Build history of the part. All positions in model axes, mm. Face numbers are marked on the shaded views. A direction names the side the tool comes from. Give positions to 0.01 mm unless a question says otherwise; leave off trailing zeros. Loops run counter-clockwise (first coordinate to the right, second up) from the corner with the lowest first, then second, coordinate; pieces in that order, holes last. Notation, with made-up numbers: (58, 38.5) -> (88, 38.5) arc R12 cw to (88, 43.5) -> close; hole circle Ø6 at (50.5, 82.5). An arc over 180 degrees is marked (long way). One line per question, with ' | ' between items. Start each with the question number.
(1) Slice it at A-A, the plane y = 0. Write the cut outline in (x, z), then the cut area to 4 significant figures.
(2) Slice it at C-C, the plane y = -3.75. Write the cut outline in (x, z), then the cut area to 4 significant figures.
(3) Flat gauge pins, fed straight in: pin 1 Ø3 at (y, z) = (0.5, 6) entering from -X; pin 2 Ø5.5 at (x, y) = (0, 0) entering from +Z; pin 3 Ø5 at (x, z) = (3.5, 12) entering from +Y; pin 4 Ø4 at (x, y) = (-3, 2) entering from +Z. Where does each tip first touch, or does it go through?
(4) Slice it at D-D, the plane z = 12.75. Write the cut outline in (x, y).
(5) Drill centre lines: L1, parallel to Y at x = 0, z = 0.35; L2, parallel to X at y = -4, z = 10.5; L3, parallel to Z at x = 3.5, y = 4.25. Where is each one in solid material? Low to high. Write a range as from..to.
(6) Mould opens along Y. For the marked faces 3, 4 and 5 say: pulls with the +Y half, pulls with the -Y half, needs draft (parallel to the pull), parting line crosses it, or undercut.
(7) 3-axis set-ups, long thin cutter, end or side, ignore diameter. For the marked faces 1 and 2: which of +Z, -Z, +X, -X, +Y, -Y reach the whole face in a straight line?
(8) Slice it at B-B, the plane x = 2. Write the cut outline in (y, z).
```python
from build123d import *

# Parameters (mm, degrees)
SKETCH1_W           = 10.5
SKETCH1_H           = 9.235397934
SKETCH1_R           = 3.5
BOSS_EXTRUDE1_DEPTH = 1.5
SKETCH1_3_W         = 1.5
SKETCH1_3_H         = 9.235397934
BOSS_EXTRUDE2_DEPTH = 15


with BuildPart() as part:
    # Sketch1 → Boss-Extrude1 (new body)
    with BuildSketch(Plane.XY):
        with Locations((-0.75, 0)):
            Rectangle(SKETCH1_W, SKETCH1_H)
        Circle(SKETCH1_R, mode=Mode.SUBTRACT)
    extrude(amount=BOSS_EXTRUDE1_DEPTH)

    # Sketch1<3> → Boss-Extrude2 (add)
    with BuildSketch(Plane.XY):
        with Locations((5.25, 0)):
            Rectangle(SKETCH1_3_W, SKETCH1_3_H)
    extrude(amount=BOSS_EXTRUDE2_DEPTH)


solid = part.part
```
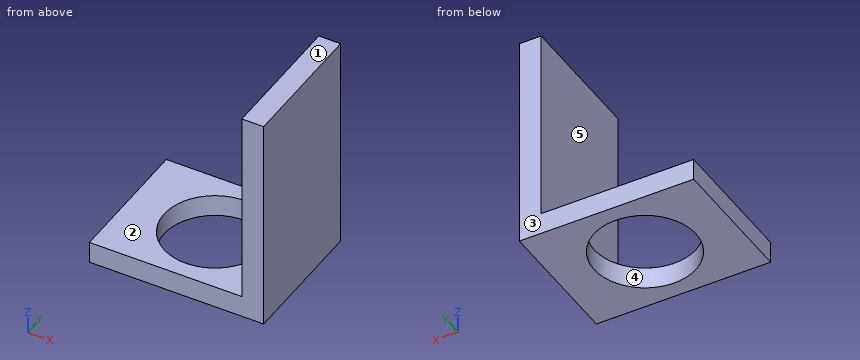
Final values:
1) outline: (-6, 0) -> (-3.5, 0) -> (-3.5, 1.5) -> (-6, 1.5) -> close; (3.5, 0) -> (6, 0) -> (6, 15) -> (4.5, 15) -> (4.5, 1.5) -> (3.5, 1.5) -> close | area: 27.75 mm2
2) outline: (-6, 0) -> (6, 0) -> (6, 15) -> (4.5, 15) -> (4.5, 1.5) -> (-6, 1.5) -> close | area: 38.25 mm2
3) pin 1: x = 4.5 | pin 2: through | pin 3: y = 4.62 | pin 4: z = 1.5
4) outline: (4.5, -4.62) -> (6, -4.62) -> (6, 4.62) -> (4.5, 4.62) -> close
5) L1: -4.62..-3.5, 3.5..4.62 | L2: 4.5..6 | L3: 0..1.5
6) face 3: pulls with the +Y half | face 4: undercut | face 5: needs draft
7) face 1: +Z, +X, -X, +Y, -Y | face 2: +Z, -X, +Y, -Y
8) outline: (-4.62, 0) -> (-2.87, 0) -> (-2.87, 1.5) -> (-4.62, 1.5) -> close; (2.87, 0) -> (4.62, 0) -> (4.62, 1.5) -> (2.87, 1.5) -> close
